Source: CAD feature listing. Evaluate the final solid. Frame: model axes, mm. Give positions to 0.01 mm unless a question says otherwise; leave off trailing zeros. Loops run counter-clockwise (first coordinate to the right, second up) from the corner with the lowest first, then second, coordinate; pieces in that order, holes last. Notation, with made-up numbers: (-6, -26.5) -> (4, -26.5) arc R27 ccw to (4, 10.5) -> close; hole circle Ø8 at (-38, -38). An arc over 180 degrees is marked (long way). Return JSON: item names as keys, results as strings. Group by question number.
(1) Ray query, line 1 (Y direction, x = 7.25, z = 0); line 2 (Y direction, x = 6.25, z = 0); line 3 (Z direction, x = 2.5, y = -29.5). Return the intervals inside material, ascending. Write a range as from..to.
(2) Pin query (flat end, axial travel): pin 1 (4 mm diameter, centred on x = 9, z = 19.5, fed in from +Y); pin 2 (3 mm diameter, centred on x = 6.5, y = -25, fed in from -Z); pin 3 (6 mm diameter, centred on x = 3.5, y = -15, fed in from -Z). Return the tip coordinate at first contact, or that it passes through.
(3) Cut plane C-C on x = 4.75. Return loops of the section in (y, z), then the cut area to 3 significant figures.
(4) Cut plane A-A on z = 0. Return loops of the section in (x, y), then the cut area to 3 significant figures.
```python
from build123d import *


with BuildPart() as part:
    # 草图1 → 旋转1 (revolve)
    with BuildSketch(Plane.XY, mode=Mode.PRIVATE) as revolve_1_sk:
        with BuildLine():
            Line((0, 35.85), (0, 33.1))
            ThreePointArc((0, 33.1), (0.175735931, 32.675735931), (0.6, 32.5))
            Line((0.6, 32.5), (9.4, 32.5))
            ThreePointArc((9.4, 32.5), (9.824264069, 32.675735931), (10, 33.1))
            Line((10, 33.1), (10, 35.85))
            Line((10, 35.85), (7.23490134, 35.85))
            ThreePointArc((7.23490134, 35.85), (5, 34.722), (2.76509866, 35.85))
            Line((2.76509866, 35.85), (0, 35.85))
        make_face()
    revolve(revolve_1_sk.sketch.rotate(Axis((-0.001266185, 0, 0), (1, 0, 0)), 270), axis=Axis((-0.001266185, 0, 0), (1, 0, 0)))


solid = part.part
```
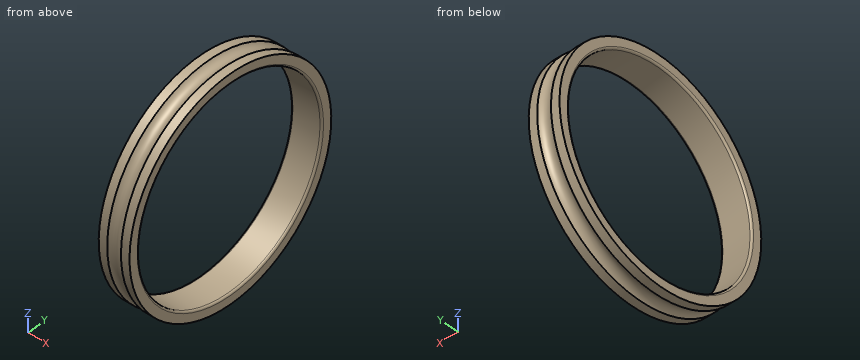
Answers:
{
 "1": {"line 1": "-35.85..-32.5, 32.5..35.85", "line 2": "-35.02..-32.5, 32.5..35.02", "line 3": "-20.37..-13.64, 13.64..20.37"},
 "2": {"pin 1": "y = 31.29", "pin 2": "z = -26.91", "pin 3": "z = -33.75"},
 "3": {"outline": "circle Ø69.47 at (0, 0); hole circle Ø65 at (0, 0)", "area": "472 mm²"},
 "4": {"outline": "(0, -35.85) -> (2.77, -35.85) arc R2.78 cw to (7.23, -35.85) -> (10, -35.85) -> (10, -33.1) arc R0.6 ccw to (9.4, -32.5) -> (0.6, -32.5) arc R0.6 ccw to (0, -33.1) -> close; (0, 33.1) arc R0.6 ccw to (0.6, 32.5) -> (9.4, 32.5) arc R0.6 ccw to (10, 33.1) -> (10, 35.85) -> (7.23, 35.85) arc R2.78 cw to (2.77, 35.85) -> (0, 35.85) -> close", "area": "59.6 mm²"}
}
